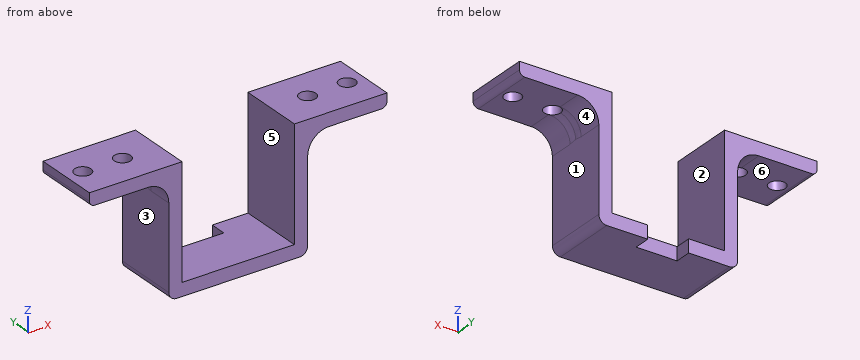
Autodesk Fusion 360 part; units mm, degrees
sketch "Sketch1" plane through (0, 0, 0) normal (0, 1, 0) x (1, 0, 0)
  line L0 (21.25, -21.25) -> (-21.25, -21.25)
  line L1 (-21.25, -21.25) -> (-21.25, 21.25)
  line L2 (-21.25, 21.25) -> (21.25, 21.25)
  line L3 (21.25, 21.25) -> (21.25, -21.25)
  line L4 (21.25, -21.25) -> (-21.25, 21.25) construction
  line L5 (-21.25, -21.25) -> (21.25, 21.25) construction
  line L6 (-21.25, -21.25) -> (-56.25, -21.25)
  line L7 (-56.25, -21.25) -> (-56.25, -16.25)
  line L8 (-56.25, -16.25) -> (-21.25, -16.25)
  line L9 (0, -21.25) -> (0, -35)
  line L10 (-26.25, -21.25) -> (-26.25, 26.25)
  line L11 (-26.25, 26.25) -> (26.25, 26.25)
  line L12 (26.25, 26.25) -> (26.25, -21.25)
  line L13 (56.25, -16.25) -> (21.25, -16.25)
  line L14 (21.25, -21.25) -> (56.25, -21.25)
  line L15 (56.25, -21.25) -> (56.25, -16.25)
  dimension "d1" = 42.5
  dimension "d2" = 42.5
  dimension "d3" = 35
  dimension "d4" = 5
extrude "Extrude1" add sketch "Sketch1" along normal blind 25 contours L3 L12 L13 L14 | L1 L2 L3 L8 L10 L11 L12 L13 | L12 L13 L14 L15 | L1 L6 L8 L10 | L6 L7 L8 L10
sketch "Sketch2" plane through (0, 0, 16.25) normal (0, 0, -1) x (-1, 0, 0)
  line L0 (26.25, 0) -> (56.25, 0)
  line L1 (56.25, 0) -> (56.25, 25)
  line L2 (56.25, 25) -> (26.25, 25)
  line L3 (26.25, 25) -> (26.25, 0)
  line L4 (0, 12.5) -> (0, 7)
  circle A0 centre (50, 12.5) radius 3.1
  circle A1 centre (35, 12.5) radius 3.1
  circle A2 centre (-35, 12.5) radius 3.1
  circle A3 centre (-50, 12.5) radius 3.1
  line L5 (0, 25) -> (7.75, 25)
  line L6 (0, 18.75) -> (7.75, 18.75)
  line L7 (7.75, 18.75) -> (7.75, 25)
  line L8 (0, 18.75) -> (-7.75, 18.75)
  line L9 (-7.75, 18.75) -> (-7.75, 25)
  line L10 (0, 25) -> (-7.75, 25)
  point P0 (0, 12.5)
  dimension "d8" = 6.2
  dimension "d9" = 6.2
  dimension "d10" = 7.75
extrude "Extrude2" cut sketch "Sketch2" along normal mid plane 144 contours A0 | A1 | A2 | A3 | L5 L6 L7 L8 L9 L10
fillet "Fillet1" radius 8 2 edges at (-26.25, 12.5, 16.25) (26.25, 12.5, 16.25)
fillet "Fillet2" radius 3 2 edges at (-26.25, 12.5, -26.25) (26.25, 12.5, -26.25)
fillet "Fillet3" radius 2 2 edges at (-56.25, 12.5, 16.25) (56.25, 12.5, 16.25)
Work out the finished part from the listing and answer in its coordinate system (mm). Face numbers are marked on the shaded views. A direction names the side the tool comes from. Give positions to 0.01 mm unless a question says otherwise; leave off trailing zeros. Order: outer loops, then holes, each group sorted by start corner. A loop starts at its lowest first (then second) coordinate and runs counter-clockwise, first axis right, second up. Notation, with made-up numbers: (-38, -2) -> (-3, -2) arc R26 cw to (-3, 30) -> close; hole circle Ø8 at (17, 1). An arc over 180 degrees is marked (long way). Answer as CSV lines item,"result". Start each with the question number.
(1) Consider line 1 along X through (y, z) = (4, 3); line 2 along Y through (x, z) = (50, 19); line 3 along Z through (x, y) = (-4, 4). Determine where each line is inside the solid, lowest interval first.
(2) Section A-A, the plane z = -15 is taken. Write down the section's boundary in (x, y), plus the area to 3 significant figures.
(3) Which of the six approach directions +Z, -Z, +X, -X, +Y, -Y give full straight-line access (tool end or side, diameter ignored) to the marked faces 1, 2 and 3?
(4) Section D-D, the plane y = 7.25 is taken. Write down the section's boundary in (x, z), plus the area to 3 significant figures.
(5) Section C-C, the plane y = 21.5 is taken. Write down the section's boundary in (x, z), plus the area to 3 significant figures.
(6) Section B-B, the plane x = -50 is taken. Write down the section's boundary in (y, z).
(7) Each of these flat-tipped pins is pushed along its axis until it touches: pin 1 Ø12.5 at (y, z) = (14, -2) entering from +X; pin 2 Ø2.5 at (y, z) = (22, -25) entering from -X; pin 3 Ø12.5 at (x, y) = (-0.5, 13.5) entering from +Z. Where does it stop, or does it pass through?
(8) For a pull along X with two mould halves and no side action, classify the marked faces 4, 5 and 6 as released by +X, released by -X, zero draft, split by the parting line, or undercut.
Entries:
1,line 1,"-26.25 to -21.25, 21.25 to 26.25"
1,line 2,"0 to 9.4, 15.6 to 25"
1,line 3,"-26.25 to -21.25"
2,outline,"(-26.25, 0) -> (-21.25, 0) -> (-21.25, 25) -> (-26.25, 25) -> close; (21.25, 0) -> (26.25, 0) -> (26.25, 25) -> (21.25, 25) -> close"
2,area,"250 mm²"
3,face 1,"-Z, +X, +Y, -Y"
3,face 2,"+Z, +Y, -Y"
3,face 3,"-Z, -X, +Y, -Y"
4,outline,"(-56.25, 18.25) arc R2 ccw to (-54.25, 16.25) -> (-34.25, 16.25) arc R8 cw to (-26.25, 8.25) -> (-26.25, -23.25) arc R3 ccw to (-23.25, -26.25) -> (23.25, -26.25) arc R3 ccw to (26.25, -23.25) -> (26.25, 8.25) arc R8 cw to (34.25, 16.25) -> (54.25, 16.25) arc R2 ccw to (56.25, 18.25) -> (56.25, 21.25) -> (21.25, 21.25) -> (21.25, -21.25) -> (-21.25, -21.25) -> (-21.25, 21.25) -> (-56.25, 21.25) -> close"
4,area,"1,010 mm²"
5,outline,"(-56.25, 18.25) arc R2 ccw to (-54.25, 16.25) -> (-34.25, 16.25) arc R8 cw to (-26.25, 8.25) -> (-26.25, -23.25) arc R3 ccw to (-23.25, -26.25) -> (-7.75, -26.25) -> (-7.75, -21.25) -> (-21.25, -21.25) -> (-21.25, 21.25) -> (-56.25, 21.25) -> close; (7.75, -26.25) -> (23.25, -26.25) arc R3 ccw to (26.25, -23.25) -> (26.25, 8.25) arc R8 cw to (34.25, 16.25) -> (54.25, 16.25) arc R2 ccw to (56.25, 18.25) -> (56.25, 21.25) -> (21.25, 21.25) -> (21.25, -21.25) -> (7.75, -21.25) -> close"
5,area,"932 mm²"
6,outline,"(0, 16.25) -> (9.4, 16.25) -> (9.4, 21.25) -> (0, 21.25) -> close; (15.6, 16.25) -> (25, 16.25) -> (25, 21.25) -> (15.6, 21.25) -> close"
7,pin 1,"x = 26.25"
7,pin 2,"x = -26.21"
7,pin 3,"z = -21.25"
8,face 4,"released by +X"
8,face 5,"undercut"
8,face 6,"zero draft"
